CAD build for the part. Positions are in the model's coordinates, mm. Face numbers are marked on the shaded views. Coordinates: 2 decimals unless noted, no trailing zeros. Write each loop counter-clockwise with the first axis right and the second up, starting at its lowest first coordinate (ties: lowest second). Pieces come first, ordered by that corner, then holes. Notation, with made-up numbers: (19.25, 83) - (47.25, 83) arc R28 ccw to (47.25, 120) - close; hole circle Ø2 at (80, 89). An arc over 180 degrees is marked (long way). One line per question, with ' | ' between items. Start each with the question number.
1. Band-saw the part on C-C, the plane z = 15.24. Write the cut outline in (x, y), then the cut area to 3 significant figures.
2. Band-saw the part on B-B, the plane z = 0. Write the cut outline in (x, y).
3. Probe line 1 (X direction, y = 5.25, z = 0); line 2 (X direction, y = 5.75, z = 15.24); line 3 (X direction, y = 6.5, z = 16.5). List the from-to ranges inside material, lowest first.
4. Band-saw the part on A-A, the plane x = 0. Write the cut outline in (y, z), then the cut area to 3 significant figures.
5. Band-saw the part on D-D, the plane y = 2.5. Write the cut outline in (x, z), then the cut area to 3 significant figures.
6. Flat gauge pin, fed straight in: P1, Ø3, axis at x = -26.4, z = 15.24, coming from the +Y side. Where does the tip first touch, or does it go through?
7. Two-plate mould, pull along Z, no slides. Class the marked faces 1, 2 and 3: +Z half, -Z half, draft (parallel to the pull), parting line (faces both ways), or undercut.
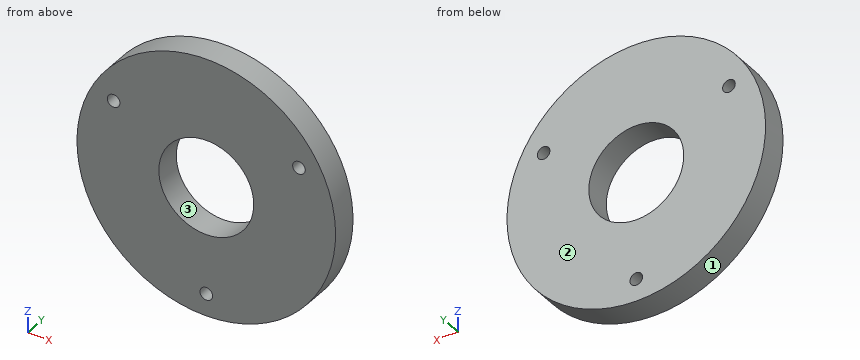
from build123d import *

# Parameters (mm, degrees)
SKETCH1_R            = 36.83
SKETCH1_R_2          = 13.5255
BOSS_EXTRUDE1_DEPTH  = 7.62
M3_CLEARANCE_HOLE1_D = 3.6


with BuildPart() as part:
    # Sketch1 → Boss-Extrude1 (new body)
    with BuildSketch(Plane(origin=(0, 0, 0), x_dir=(1, 0, 0), z_dir=(0, 1, 0))):
        with Locations(Location((0, 0, 0), (0, 0, 90))):
            Circle(SKETCH1_R)
        with Locations(Location((0, 0, 0), (0, 0, 90))):
            Circle(SKETCH1_R_2, mode=Mode.SUBTRACT)
    extrude(amount=BOSS_EXTRUDE1_DEPTH)

    # M3 Clearance Hole1 (through all)
    with Locations(Plane(origin=(0, 7.62, 0), x_dir=(1, 0, 0), z_dir=(0, 1, 0))):
        with Locations((0, 30.48), (26.396454307, -15.24), (-26.396454307, -15.24)):
            Hole(M3_CLEARANCE_HOLE1_D / 2)


solid = part.part
Filled in:
1) outline: (-33.53, 0) - (-28.2, 0) - (-28.2, 7.62) - (-33.53, 7.62) - close; (-24.6, 0) - (24.6, 0) - (24.6, 7.62) - (-24.6, 7.62) - close; (28.2, 0) - (33.53, 0) - (33.53, 7.62) - (28.2, 7.62) - close | area: 456 mm²
2) outline: (-36.83, 0) - (-13.53, 0) - (-13.53, 7.62) - (-36.83, 7.62) - close; (13.53, 0) - (36.83, 0) - (36.83, 7.62) - (13.53, 7.62) - close
3) line 1: x = -36.83 to -13.53, 13.53 to 36.83 | line 2: x = -33.53 to -28.2, -24.6 to 24.6, 28.2 to 33.53 | line 3: x = -32.93 to -27.68, -25.11 to 25.11, 27.68 to 32.93
4) outline: (0, -36.83) - (7.62, -36.83) - (7.62, -32.28) - (0, -32.28) - close; (0, -28.68) - (7.62, -28.68) - (7.62, -13.53) - (0, -13.53) - close; (0, 13.53) - (7.62, 13.53) - (7.62, 36.83) - (0, 36.83) - close | area: 328 mm²
5) outline: circle Ø73.66 at (0, 0); hole circle Ø3.6 at (-26.4, 15.24); hole circle Ø27.05 at (0, 0); hole circle Ø3.6 at (0, -30.48); hole circle Ø3.6 at (26.4, 15.24) | area: 3,660 mm²
6) P1: passes through
7) face 1: parting line | face 2: draft | face 3: undercut
